Part model, mm, in its own coordinate system. A direction names the side the tool comes from. Give positions to 0.01 mm unless a question says otherwise; leave off trailing zeros. Order: outer loops, then holes, each group sorted by start corner. A loop starts at its lowest first (then second) coordinate and runs counter-clockwise, first axis right, second up. Notation, with made-up numbers: M 8.25,-26.5 L 19.25,-26.5 A27 ccw 19.25,-4.5 Z; hole C -36,72.5 d10. An arc over 180 degrees is marked long. Return JSON: item names as keys, results as strings.
Autodesk Inventor part; units mm, degrees
ref_plane "YZ Plane" through (0, 0, 0) normal (1, 0, 0) x (0, 1, 0)
ref_plane "XZ Plane" through (0, 0, 0) normal (0, 1, 0) x (-1, 0, 0)
ref_plane "XY Plane" through (0, 0, 0) normal (0, 0, 1) x (1, 0, 0)
sketch "スケッチ1" plane through (0, 0, 0) normal (0, 0, 1) x (1, 0, 0)
  circle A0 centre (0, 0) radius 14.5
  dimension "d0" = 29
extrude "押し出し1" add sketch "スケッチ1" along normal blind 50
sketch "スケッチ2" plane through (0, 0, 50) normal (0, 0, 1) x (1, 0, 0)
  circle A0 centre (0, 0) radius 5
  dimension "d3" = 10
extrude "押し出し2" add sketch "スケッチ2" along normal blind 2.7
sketch "スケッチ3" plane through (0, 0, 52.7) normal (0, 0, 1) x (1, 0, 0)
  circle A0 centre (0, 0) radius 1.25
  dimension "d6" = 2.5
extrude "押し出し3" add sketch "スケッチ3" along normal blind 9.3
sketch "スケッチ4" plane through (0, 0, 50) normal (0, 0, 1) x (1, 0, 0)
  circle A0 centre (0, 0) radius 14.5
  line L0 (0, 14.5) -> (0, -14.5)
  point P0 (-8, 0)
  point P1 (8, 0)
  dimension "d9" = 16
hole "穴1" at (-8, 0, 50) at (8, 0, 50) direction (0, 0, -1) diameter 2.1129 depth 3 tip angle 118
properties part number "RD008"
Q1. Band-saw the part on C-C (z = 38). Give the cut face in (x, y), then the cut area to 3 significant figures.
Established:
{"outline": "C 0,0 d29", "area": "661 mm²"}
Q2. Probe line 1 along Z through (x, y) = (10.75, 3); line 2 along Y through (x, z) = (-8, 49.2); line 3 along Y through (x, z) = (-2, 25.5). List the from-to ranges inside material, lowest first.
Established:
{"line 1": "z = 0 to 50", "line 2": "y = -12.09 to -1.06, 1.06 to 12.09", "line 3": "y = -14.36 to 14.36"}
Q3. Band-saw the part on D-D (y = 3.5). Give the cut face in (x, z), then the cut area to 3 significant figures.
Established:
{"outline": "M -14.07,0 L 14.07,0 L 14.07,50 L 3.57,50 L 3.57,52.7 L -3.57,52.7 L -3.57,50 L -14.07,50 Z", "area": "1,430 mm²"}
Q4. Pin check, flat tips, straight feed: pin 1 (1.7 mm diameter, centred on x = 8, y = 0, fed in from +Z); pin 2 (3 mm diameter, centred on x = 9, z = 43.5, fed in from +Y); pin 3 (1.5 mm diameter, centred on x = -10.5, z = 25, fed in from +Y). Stop position of each tip, or through.
Established:
{"pin 1": "stops at z = 46.88", "pin 2": "stops at y = 12.41", "pin 3": "stops at y = 10.73"}
Q5. Band-saw the part on A-A (x = 0). Give the cut face in (y, z), then the cut area to 3 significant figures.
Established:
{"outline": "M -14.5,0 L 14.5,0 L 14.5,50 L 5,50 L 5,52.7 L 1.25,52.7 L 1.25,62 L -1.25,62 L -1.25,52.7 L -5,52.7 L -5,50 L -14.5,50 Z", "area": "1,500 mm²"}
Q6. Band-saw the part on B-B (y = -2). Give the cut face in (x, z), then the cut area to 3 significant figures.
Established:
{"outline": "M -14.36,0 L 14.36,0 L 14.36,50 L 4.58,50 L 4.58,52.7 L -4.58,52.7 L -4.58,50 L -14.36,50 Z", "area": "1,460 mm²"}
Q7. Two-plate mould, pull along Y, no slides. Class faces 3 (the cylindrical face through (-6.97, 0.23, 48.48)), 4 (the flat face through (6, 0, 50)), 5 (the cylindrical face through (6.691, 12.864, 24.65)): +Y half, -Y half, draft (parallel to the pull), parting line (faces both ways), or undercut.
Established:
{"face 3": "undercut", "face 4": "draft", "face 5": "parting line"}
Q8. 3-axis set-ups, long thin cutter, end or side, ignore diameter. For faces 1 (the flat face through (0, 0, 0)), 2 (the cylindrical face through (-1.08, 4.88, 51.33)): which of +Z, -Z, +X, -X, +Y, -Y reach the whole face in a straight line?
Established:
{"face 1": "-Z, +X, -X, +Y, -Y", "face 2": "+Z"}
